Source: CAD feature listing. Evaluate the final solid. Frame: model axes, mm. A direction names the side the tool comes from. Give positions to 0.01 mm unless a question says otherwise; leave off trailing zeros. Loops run counter-clockwise (first coordinate to the right, second up) from the corner with the lowest first, then second, coordinate; pieces in that order, holes last. Notation, with made-up numbers: M 0,-28.5 L 58,-28.5 A17 cw 58,-3.5 Z; hole C 55,85 d7. An arc over 180 degrees is marked long. Answer in a Markdown table with one row per item.
```python
from build123d import *

# Parameters (mm, degrees)
SKETCH_R          = 4
PAD_DEPTH         = 110
SKETCH001_R       = 11.25
PAD001_DEPTH      = 70
PAD001_DEPTH_BACK = 75
SKETCH003_R       = 8
PAD002_DEPTH      = 90
POCKET_DEPTH      = 18


with BuildPart() as part:
    # Sketch → Pad (new body)
    with BuildSketch(Plane.YZ):
        Circle(SKETCH_R)
    extrude(amount=-PAD_DEPTH)

    # Sketch001 → Pad001 (join, two sides)
    with BuildSketch(Plane.YZ) as pad001_sk:
        Circle(SKETCH001_R)
    extrude(amount=PAD001_DEPTH)
    extrude(pad001_sk.sketch, amount=-PAD001_DEPTH_BACK)

    # Sketch003 → Pad002 (join)
    with BuildSketch(Plane.YZ):
        Circle(SKETCH003_R)
    extrude(amount=PAD002_DEPTH)

    # Sketch002 → Pocket (cut)
    with BuildSketch(Plane.YZ.offset(90)):
        with BuildLine():
            ThreePointArc((2.99806, -0.107877), (-1.918287, 2.306551), (-0.44036, -2.967505))
            Line((-0.44036, -2.967505), (0.198883, -3.73651))
            Line((0.198883, -3.73651), (3.637995, -0.877715))
            Line((2.99806, -0.107877), (3.637995, -0.877715))
        make_face()
    extrude(amount=-POCKET_DEPTH, mode=Mode.SUBTRACT)


solid = part.part
```
Q1. Section query C-C (x = 11). Output: boundary loops of the cut face in (y, z).
Values follow:
| item | result |
|---|---|
| outline | C 0,0 d22.5 |
Q2. Section query A-A (x = -89.5). Output: boundary loops of the cut face in (y, z), plus the area to 3 significant figures.
Values follow:
| item | result |
|---|---|
| outline | C 0,0 d8 |
| area | 50.3 mm^2 |
Q3. Reachability of faces 1 (the flat face through (90, 3.4, 0.1)), 2 (the flat face through (-75, 5, 0)), 3 (the cylindrical face through (81.1, -1.8, 2.4)) from +Z, -Z, +X, -X, +Y, -Y: full face, straight path, thin tool, end or side. Return the list, or none.
Values follow:
| item | result |
|---|---|
| face 1 | +Z, -Z, +X, +Y, -Y |
| face 2 | -X |
| face 3 | +X |
Q4. Mould query, pull axis Z, two halves, no side actions, for faces 4 (the cylindrical face through (-1.48, 5.19, -9.98)), 5 (the flat face through (70, 2, 8)), 6 (the flat face through (72, 0, 0)). Classes: +Z half, -Z half, draft (parallel to the pull), parting line (faces both ways), or undercut.
Values follow:
| item | result |
|---|---|
| face 4 | parting line |
| face 5 | draft |
| face 6 | undercut |
Q5. Section query B-B (z = 6). Output: boundary loops of the cut face in (x, y), plus the area to 3 significant figures.
Values follow:
| item | result |
|---|---|
| outline | M -75,-9.52 L 70,-9.52 L 70,-5.29 L 90,-5.29 L 90,5.29 L 70,5.29 L 70,9.52 L -75,9.52 Z |
| area | 2,970 mm^2 |
Q6. Contact query for flat-ended pins moving along their axis: pin 1 Ø5 at (y, z) = (-7, -8) entering from +X; pin 2 Ø11 at (y, z) = (-3, 4.5) entering from -X; pin 3 Ø12 at (x, y) = (-74.5, 8.5) entering from -Z; pin 4 Ø5 at (x, z) = (-48.5, -7.5) entering from +Y. Output: stop coordinate, or through.
Values follow:
| item | result |
|---|---|
| pin 1 | x = 70 |
| pin 2 | x = -110 |
| pin 3 | z = -10.97 |
| pin 4 | y = 10.08 |
Q7. Ray query, probe 1 along Y at (x, z) = (78.75, 0); probe 2 along X at (y, z) = (-4.5, -4.5); probe 3 along X at (y, z) = (-9, 5.5). Return the intervals inside material, ascending. Write a range as from..to.
Values follow:
| item | result |
|---|---|
| probe 1 | -8..-3, 3..8 |
| probe 2 | -75..90 |
| probe 3 | -75..70 |
